Autodesk Inventor part; units mm, degrees
ref_plane "YZ Plane" through (0, 0, 0) normal (1, 0, 0) x (0, 1, 0)
ref_plane "XZ Plane" through (0, 0, 0) normal (0, 1, 0) x (-1, 0, 0)
ref_plane "XY Plane" through (0, 0, 0) normal (0, 0, 1) x (1, 0, 0)
sketch "Sketch1" plane through (0, 0, 0) normal (0, 0, 1) x (1, 0, 0)
  line L0 (0, 0) -> (50, 0)
  line L1 (50, 0) -> (50, 52.5)
  line L2 (50, 52.5) -> (0, 52.5)
  line L3 (0, 52.5) -> (0, 0)
  dimension "d0" = 50
  dimension "d1" = 52.5
extrude "Extrusion1" add sketch "Sketch1" along normal blind 2
sketch "Sketch2" plane through (0, 0, 2) normal (0, 0, 1) x (1, 0, 0)
  line L0 (2, 50.5) -> (48, 50.5)
  line L1 (48, 50.5) -> (48, 2)
  line L2 (48, 2) -> (2, 2)
  line L3 (2, 2) -> (2, 50.5)
  dimension "d4" = 46
  dimension "d5" = 48.5
extrude "Extrusion2" cut sketch "Sketch2" against normal blind 10
sketch "Sketch3" plane through (0, 0, 0) normal (-1, 0, 0) x (0, 0, 1)
  line L0 (0, 52.5) -> (0, 0)
  line L1 (0, 0) -> (2, 0)
  line L2 (2, 52.5) -> (2, 0)
  line L3 (0, 52.5) -> (2, 52.5)
extrude "Extrusion3" add sketch "Sketch3" along normal blind 8.5
sketch "Sketch4" plane through (50, 0, 0) normal (1, 0, 0) x (0, 0, -1)
  line L0 (0, 0) -> (0, 52.5)
  line L1 (0, 52.5) -> (-2, 52.5)
  line L2 (-2, 0) -> (-2, 52.5)
  line L3 (0, 0) -> (-2, 0)
extrude "Extrusion4" add sketch "Sketch4" along normal blind 2
properties part number "Zijplaat 2"
The model under review builds one solid part; all positions refer to its coordinate system, in mm. A direction names the side the tool comes from. Round coordinates to 2 decimals unless told otherwise and drop trailing zeros. Loops run counter-clockwise (first coordinate to the right, second up) from the corner with the lowest first, then second, coordinate; pieces in that order, holes last. Notation, with made-up numbers: (22, -37) -> (38, -37) arc R21 ccw to (38, -13) -> close; hole circle Ø1 at (76.25, 19.5). An arc over 180 degrees is marked (long way). One line per question, with ' | ' between items. Start each with the question number.
Item 1: Add section A-A, the plane x = 24. Write out the cut boundary in (y, z), then the cut area to 3 significant figures.
Item 2: Add section B-B, the plane y = 42.5. Write out the cut boundary in (x, z), then the cut area to 3 significant figures.
Item 3: Machinability: for faces 5 (the face through (25, 2, 1)), 6 (the face through (-8.5, 27, 1)), which of the approach directions +Z, -Z, +X, -X, +Y, -Y give a long, thin tool a straight path to every point of the face, cutting with its end or side? Answer none if there is none.
Item 4: Add section C-C, the plane z = 1.05. Write out the cut boundary in (x, y).
Item 5: Draft analysis for pull direction Y (two halves, no side actions). For faces 1 (the face through (52, 27, 1)), 2 (the face through (21, 0, 1)), 3 (the face through (21, 52.5, 1)), 4 (the face through (48, 27, 1)), state which applies: +Y half, -Y half, draft (parallel to the pull), parting line (faces both ways), or undercut.
Item 6: For pin 1 (0.6 mm diameter, centred on x = 24.5, z = 0.5, fed in from -Y), flat-tipped, find the tip position at first contact; note if it passes through.
Item 7: Wall thickness on line 1 along X through (y, z) = (28, 1.5); line 2 along Y through (x, z) = (6, 1.95): over which ranges is each line inside the solid? List them lowest first. Write a range as [from, to].
Return value:
1) outline: (0, 0) -> (2, 0) -> (2, 2) -> (0, 2) -> close; (50.5, 0) -> (52.5, 0) -> (52.5, 2) -> (50.5, 2) -> close | area: 8.00 mm2
2) outline: (-8.5, 0) -> (2, 0) -> (2, 2) -> (-8.5, 2) -> close; (48, 0) -> (52, 0) -> (52, 2) -> (48, 2) -> close | area: 29.0 mm2
3) face 5: +Z, -Z | face 6: +Z, -Z, -X, +Y, -Y
4) outline: (-8.5, 0) -> (52, 0) -> (52, 52.5) -> (-8.5, 52.5) -> close; hole (2, 2) -> (48, 2) -> (48, 50.5) -> (2, 50.5) -> close
5) face 1: draft | face 2: -Y half | face 3: +Y half | face 4: undercut
6) pin 1: stops at y = 0
7) line 1: x = [-8.5, 2], [48, 52] | line 2: y = [0, 2], [50.5, 52.5]
